from build123d import *

# Parameters (mm, degrees)
BOSS_EXTRUDE1_DEPTH     = 5
SKETCH4_W               = 2
SKETCH4_H               = 8
BOSS_EXTRUDE2_DEPTH     = 12
SKETCH5_R               = 2.5
CUT_EXTRUDE1_DEPTH      = 51
CUT_EXTRUDE1_DEPTH_BACK = 51


with BuildPart() as part:
    # Sketch2 → Boss-Extrude1 (new body)
    with BuildSketch(Plane.XY):
        with BuildLine():
            Line((-20, 80), (20, 80))
            Line((20, 80), (20, 70))
            Line((20, 70), (18, 70))
            ThreePointArc((18, 70), (10.928932188, 67.071067812), (8, 60))
            Line((8, 60), (8, 20))
            ThreePointArc((8, 20), (10.928932188, 12.928932188), (18, 10))
            Line((18, 10), (50, 10))
            Line((50, 10), (50, 0))
            Line((50, 0), (-50, 0))
            Line((-50, 0), (-50, 10))
            Line((-50, 10), (-18, 10))
            ThreePointArc((-18, 10), (-10.928932188, 12.928932188), (-8, 20))
            Line((-8, 20), (-8, 60))
            ThreePointArc((-8, 60), (-10.928932188, 67.071067812), (-18, 70))
            Line((-18, 70), (-20, 70))
            Line((-20, 70), (-20, 80))
        make_face()
    extrude(amount=BOSS_EXTRUDE1_DEPTH)

    # Sketch4 → Boss-Extrude2 (add)
    with BuildSketch(Plane.XY.offset(5)):
        with Locations((-9, 75)):
            Rectangle(SKETCH4_W, SKETCH4_H)
        with Locations((9, 75)):
            Rectangle(SKETCH4_W, SKETCH4_H)
        with Locations((-41, 5)):
            Rectangle(SKETCH4_W, SKETCH4_H)
        with Locations((-31, 5)):
            Rectangle(SKETCH4_W, SKETCH4_H)
        with Locations((31, 5)):
            Rectangle(SKETCH4_W, SKETCH4_H)
        with Locations((41, 5)):
            Rectangle(SKETCH4_W, SKETCH4_H)
    extrude(amount=BOSS_EXTRUDE2_DEPTH)

    # Sketch5 → Cut-Extrude1 (cut, two sides)
    with BuildSketch(Plane(origin=(0, 0, 0), x_dir=(0, 0, -1), z_dir=(1, 0, 0))) as cut_extrude1_sk:
        with Locations((-12, 75)):
            Circle(SKETCH5_R)
        with Locations((-12, 5)):
            Circle(SKETCH5_R)
        with BuildLine():
            Line((-12, 79), (-17, 79))
            Line((-17, 79), (-17, 71))
            Line((-17, 71), (-12, 71))
            ThreePointArc((-12, 71), (-16, 75), (-12, 79))
        make_face()
        with BuildLine():
            Line((-12, 9), (-17, 9))
            Line((-17, 9), (-17, 1))
            Line((-17, 1), (-12, 1))
            ThreePointArc((-12, 1), (-16, 5), (-12, 9))
        make_face()
    extrude(amount=CUT_EXTRUDE1_DEPTH, mode=Mode.SUBTRACT)
    extrude(cut_extrude1_sk.sketch, amount=-CUT_EXTRUDE1_DEPTH_BACK, mode=Mode.SUBTRACT)


solid = part.part
Could you check a few things on this model? Use its own coordinates, in mm. A direction names the side the tool comes from. Give positions to 0.01 mm unless a question says otherwise; leave off trailing zeros. Order: outer loops, then holes, each group sorted by start corner. A loop starts at its lowest first (then second) coordinate and runs counter-clockwise, first axis right, second up.
Item 1: If we section it at A-A, the plane z = 7: Write out the boundary of the cut face in (x, y), plus the area to 3 significant figures.
Item 2: If we section it at D-D, the plane x = -35: Write out the boundary of the cut face in (y, z), plus the area to 3 significant figures.
Item 3: If we section it at B-B, the plane y = 75: Write out the boundary of the cut face in (x, z), plus the area to 3 significant figures.
Item 4: For faces 1 (the face through (-41, 9, 8)), 2 (the face through (-9, 71, 8)), 3 (the face through (10.85, 13.01, 2.46)), 4 (the face through (20, 75, 2)), 5 (the face through (40, 5, 9)), which set-ups out of +Z, -Z, +X, -X, +Y, -Y let a thin tool reach every point of the face, with its end or its side?
Item 5: If we section it at C-C, the plane y = 5: Count the separate pieces of the cut face and the enclosed holes in it, plus the area to 3 significant figures.
Item 6: I need wall thicknesses on line 1 (Y direction, x = 40.7, z = 12); line 2 (Y direction, x = 9.2, z = 12); line 3 (Z direction, x = 41, y = 5). Which ranges of each line are inside material? Lowest first, please.
Item 7: I'm going to push flat-ended pins straight in: pin 1 (1.6 mm diameter, centred on x = 41, z = 7, fed in from +Y); pin 2 (4 mm diameter, centred on y = 4.5, z = 9, fed in from -X); pin 3 (1.5 mm diameter, centred on x = 37.5, z = 3.5, fed in from +Y). Where does each tip first touch, or does it pass through?
Item 8: If we mould it in two halves opening along Y, with no side actions, what happens to faces 6 (the face through (-11.01, 12.85, 2.46)), 7 (the face through (1, 0, 2)), 8 (the face through (30, 5, 9)), 9 (the face through (31, 9, 8))? For each: pulls with the +Y half, pulls with the -Y half, needs draft (parallel to the pull), parting line crosses it, or undercut.
Values:
1. outline: (-42, 1) - (-40, 1) - (-40, 9) - (-42, 9) - close; (-32, 1) - (-30, 1) - (-30, 9) - (-32, 9) - close; (-10, 71) - (-8, 71) - (-8, 79) - (-10, 79) - close; (8, 71) - (10, 71) - (10, 79) - (8, 79) - close; (30, 1) - (32, 1) - (32, 9) - (30, 9) - close; (40, 1) - (42, 1) - (42, 9) - (40, 9) - close
1. area: 96.0 mm2
2. outline: (0, 0) - (10, 0) - (10, 5) - (0, 5) - close
2. area: 50.0 mm2
3. outline: (-20, 0) - (20, 0) - (20, 5) - (10, 5) - (10, 9.5) - (8, 9.5) - (8, 5) - (-8, 5) - (-8, 9.5) - (-10, 9.5) - (-10, 5) - (-20, 5) - close; (-10, 14.5) - (-8, 14.5) - (-8, 16) - (-10, 16) - close; (8, 14.5) - (10, 14.5) - (10, 16) - (8, 16) - close
3. area: 224 mm2
4. face 1: +Z, +X, -X, +Y
4. face 2: +Z, +X, -X, -Y
4. face 3: +Z, -Z, +X
4. face 4: +Z, -Z, +X, +Y
4. face 5: +Z, +Y, -Y
5. separate pieces: 5
5. enclosed holes: 0
5. area: 548 mm2
6. line 1: y = 1 to 2.5, 7.5 to 9
6. line 2: y = 71 to 72.5, 77.5 to 79
6. line 3: z = 0 to 9.5, 14.5 to 16
7. pin 1: stops at y = 9
7. pin 2: stops at x = -42
7. pin 3: stops at y = 10
8. face 6: undercut
8. face 7: pulls with the -Y half
8. face 8: needs draft
8. face 9: pulls with the +Y half
